from build123d import *

# Parameters (mm, degrees)
F2_R      = 4
F3_DEPTH  = 25
F4_W      = 2.5
F4_H      = 2.5
F5_DEPTH  = 6
F6_DEPTH  = 3
F7_W      = 7.8000803478
F7_H      = 15
F8_DEPTH  = 23.7818172899
F9_DEPTH  = 25
F10_R     = 3
F11_DEPTH = 2


with BuildPart() as f1:
    # F0 (on Front) → F1 (revolve)
    with BuildSketch(Plane.XZ):
        Polygon((0, 20), (0, 0), (12, 0), align=None)
    revolve(axis=Axis((0, 0, 10), (0, 0, -1)))

    # F2 (on Top) → F3 (join)
    with BuildSketch(Plane.XY):
        Circle(F2_R)
    extrude(amount=F3_DEPTH)



with BuildPart() as f5:
    # F4 (on Front) → F5 (new body)
    with BuildSketch(Plane.XZ):
        with Locations((20.4691827101, 44.25)):
            Rectangle(F4_W, F4_H)
    extrude(amount=-F5_DEPTH)


with BuildPart() as f5b:
    # F4 (on Front) → F5, piece 2 (new body)
    with BuildSketch(Plane.XZ):
        with Locations((-22.5308172899, 26.25)):
            Rectangle(F4_W, F4_H)
    extrude(amount=-F5_DEPTH)


with BuildPart() as f5c:
    # F4 (on Front) → F5, piece 3 (new body)
    with BuildSketch(Plane.XZ):
        with Locations((-22.5308172899, 44.25)):
            Rectangle(F4_W, F4_H)
    extrude(amount=-F5_DEPTH)


with BuildPart() as f5d:
    # F4 (on Front) → F5, piece 4 (new body)
    with BuildSketch(Plane.XZ):
        with Locations((20.4691827101, 26.25)):
            Rectangle(F4_W, F4_H)
    extrude(amount=-F5_DEPTH)


with BuildPart() as f1_1:
    add(f1.part)

    add(f5.part)  # F6 merges F5

    add(f5b.part)  # F6 merges F5b

    add(f5c.part)  # F6 merges F5c

    add(f5d.part)  # F6 merges F5d
    # F4 (on Front) → F6 (join)
    with BuildSketch(Plane.XZ):
        with Locations((-22.5308172899, 44.25)):
            Rectangle(F4_W, F4_H)
        Polygon((19.2191827101, 45.5), (-21.2808172899, 45.5), (-21.2808172899, 43), (-23.7808172899, 43), (-23.7808172899, 27.5), (-21.2808172899, 27.5), (-21.2808172899, 25), (19.2191827101, 25), (19.2191827101, 27.5), (21.7191827101, 27.5), (21.7191827101, 43), (19.2191827101, 43), align=None)
        with Locations((20.4691827101, 44.25)):
            Rectangle(F4_W, F4_H)
        with Locations((-22.5308172899, 26.25)):
            Rectangle(F4_W, F4_H)
        with Locations((20.4691827101, 26.25)):
            Rectangle(F4_W, F4_H)
    extrude(amount=F6_DEPTH)

    # F7 (on Right) → F8 (cut, through all)
    with BuildSketch(Plane.YZ):
        with Locations((3.9000401739, 17.5)):
            Rectangle(F7_W, F7_H)
    extrude(amount=-F8_DEPTH, mode=Mode.SUBTRACT)

    # F7 (on Right) → F9 (cut)
    with BuildSketch(Plane.YZ):
        with Locations((3.9000401739, 17.5)):
            Rectangle(F7_W, F7_H)
    extrude(amount=F9_DEPTH, mode=Mode.SUBTRACT)

    # F10 (on Top) → F11 (cut)
    with BuildSketch(Plane.XY):
        Circle(F10_R)
    extrude(amount=F11_DEPTH, mode=Mode.SUBTRACT)


solid = f1_1.part
Verification items for the finished model (mm, model axes). A direction names the side the tool comes from. Coordinates: 2 decimals unless noted, no trailing zeros. Write each loop counter-clockwise with the first axis right and the second up, starting at its lowest first coordinate (ties: lowest second). Pieces come first, ordered by that corner, then holes. Notation, with made-up numbers: M 16.25,12 L 44.25,12 A26 ccw 44.25,38 Z; hole C -10.5,7 d5. An arc over 180 degrees is marked long. Use a Markdown table: item, result.
Q1. Draft check along Z on faces 6 (the face through (20, 3, 27.5)), 7 (the face through (20, 6, 26)), 8 (the face through (0, 2, 10)). Enter one of: +Z half, -Z half, draft (parallel to the pull), parting line (faces both ways), or undercut.
Reply:
| item | result |
|---|---|
| face 6 | undercut |
| face 7 | draft |
| face 8 | +Z half |
Q2. Sectioned sample at D-D, the plane z = 37.5. Record the boundary of the cut face in (x, y), plus the area to 4 significant figures.
Reply:
| item | result |
|---|---|
| outline | M -23.78,-3 L 21.72,-3 L 21.72,0 L -23.78,0 Z |
| area | 136.5 mm² |
Q3. Sectioned sample at A-A, the plane x = 0. Record the boundary of the cut face in (y, z).
Reply:
| item | result |
|---|---|
| outline | M -12,0 L -3,0 L -3,2 L 3,2 L 3,0 L 12,0 L 6,10 L 0,10 L 0,45.5 L -3,45.5 L -3,25 L -4,25 L -4,13.33 Z |
Q4. Go/stop test with flat-tipped pins: P1, Ø1.2, axis at x = -22.5, z = 26.5, coming from the +Y side; P2, Ø1, axis at x = -12.5, z = 38.5, coming from the +Y side; P3, Ø5, axis at y = -8.5, z = 21.5, coming from the -X side; P4, Ø16.5, axis at x = -1, z = 32, coming from the -Y side. Record where each tip stops, or that it passes through.
Reply:
| item | result |
|---|---|
| P1 | stops at y = 6 |
| P2 | stops at y = 0 |
| P3 | passes through |
| P4 | stops at y = -4 |
Q5. Sectioned sample at C-C, the plane x = -14. Record the boundary of the cut face in (y, z), plus the area to 3 significant figures.
Reply:
| item | result |
|---|---|
| outline | M -3,25 L 0,25 L 0,45.5 L -3,45.5 Z |
| area | 61.5 mm² |
Q6. Thickness scan on line 1 (Y direction, x = -3.5, z = 27); line 2 (Y direction, x = 0, z = 1); line 3 (Z direction, x = 20, y = -2.25). Record the ranges inside material, lowest first.
Reply:
| item | result |
|---|---|
| line 1 | y = -3 to 0 |
| line 2 | y = -11.4 to -3, 3 to 11.4 |
| line 3 | z = 25 to 45.5 |
Q7. Set-up check for faces 1 (the face through (-0.803, -6.114, 9.723)), 2 (the face through (20, 3, 43)), 3 (the face through (-1, -3, 35)), 4 (the face through (-21.281, 3, 26)), 5 (the face through (0, 0, 2)): record each of +Z, -Z, +X, -X, +Y, -Y from which the full face is reachable in a straight line by a thin tool's end or side.
Reply:
| item | result |
|---|---|
| face 1 | none |
| face 2 | +X, -X, +Y |
| face 3 | +Z, +X, -X, -Y |
| face 4 | +Z, -Z, +Y |
| face 5 | -Z |
Q8. Sectioned sample at B-B, the plane z = 20. Record the boundary of the cut face in (x, y), plus the area to 3 significant figures.
Reply:
| item | result |
|---|---|
| outline | M -4,0 A4 ccw 4,0 Z |
| area | 25.1 mm² |
